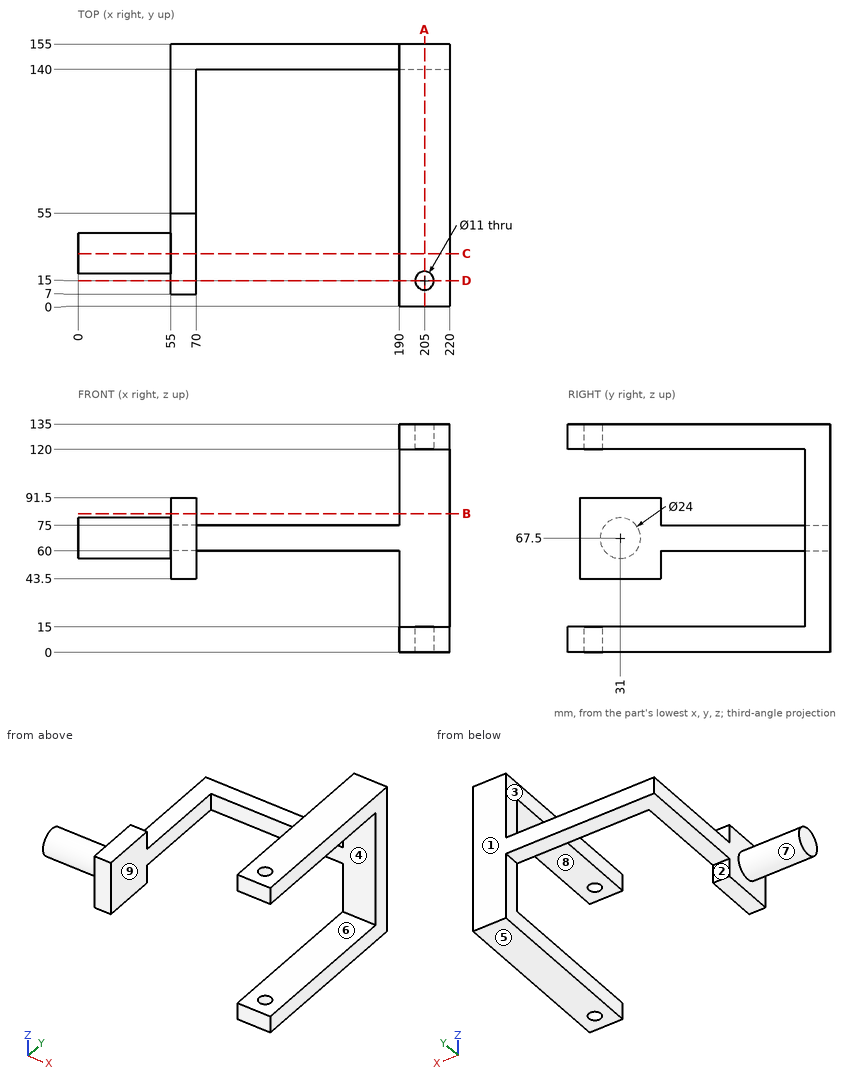
Answer from the drawing. Dimensions are ordinates in mm from the lowest x, y and z of the part. A direction names the side the tool comes from. Coordinates: 2 decimals unless noted, no trailing zeros. Loops run counter-clockwise (first coordinate to the right, second up) from the corner with the lowest first, then second, coordinate; pieces in that order, holes last. Notation, with made-up numbers: (54.25, 75.25) -> (60.25, 75.25) arc R24 cw to (60.25, 88.25) -> close; hole circle Ø11 at (-30.5, 71). An arc over 180 degrees is marked (long way). Return JSON: item names as keys, results as strings.
Item 1: Find section B-B (z = 82). Determine the outline of the cut face in (x, y), plus the area to 3 significant figures.
Answers:
{"outline": "(55, 7) -> (70, 7) -> (70, 55) -> (55, 55) -> close; (190, 140) -> (220, 140) -> (220, 155) -> (190, 155) -> close", "area": "1,170 mm2"}
Item 2: For a pull along Z with two mould halves and no side action, classify the marked faces 6, 7, 8 and 9 as +Z half, -Z half, draft (parallel to the pull), parting line (faces both ways), or undercut.
Answers:
{"face 6": "undercut", "face 7": "parting line", "face 8": "undercut", "face 9": "draft"}
Item 3: Find section D-D (y = 15). Determine the outline of the cut face in (x, z).
Answers:
{"outline": "(55, 43.5) -> (70, 43.5) -> (70, 91.5) -> (55, 91.5) -> close; (190, 0) -> (199.5, 0) -> (199.5, 15) -> (190, 15) -> close; (190, 120) -> (199.5, 120) -> (199.5, 135) -> (190, 135) -> close; (210.5, 0) -> (220, 0) -> (220, 15) -> (210.5, 15) -> close; (210.5, 120) -> (220, 120) -> (220, 135) -> (210.5, 135) -> close"}
Item 4: For the marked faces 1, 2, 3, 4 and 5, determine the directions among +Z, -Z, +X, -X, +Y, -Y from which every point of the face is accessible in a straight line to the end or side of a thin tool.
Answers:
{"face 1": "+Z, -Z, +X, -X, +Y", "face 2": "-Z, +X, -X, +Y", "face 3": "+Z, -X, +Y, -Y", "face 4": "+X, -Y", "face 5": "-Z, +X, -X, +Y, -Y"}
Item 5: Find section A-A (x = 205). Determine the outline of the cut face in (y, z).
Answers:
{"outline": "(0, 0) -> (9.5, 0) -> (9.5, 15) -> (0, 15) -> close; (0, 120) -> (9.5, 120) -> (9.5, 135) -> (0, 135) -> close; (20.5, 0) -> (155, 0) -> (155, 135) -> (20.5, 135) -> (20.5, 120) -> (140, 120) -> (140, 15) -> (20.5, 15) -> close"}
Item 6: Find the intervals of material crossed by probe 1 along Z at (x, y) = (208.5, 95.5); probe 2 along Y at (x, z) = (205, 4); probe 3 along Z at (x, y) = (103, 142), in increasing order.
Answers:
{"probe 1": "z = 0 to 15, 120 to 135", "probe 2": "y = 0 to 9.5, 20.5 to 155", "probe 3": "z = 60 to 75"}
Item 7: Find section C-C (y = 31). Determine the outline of the cut face in (x, z), plus the area to 3 significant figures.
Answers:
{"outline": "(0, 55.5) -> (55, 55.5) -> (55, 43.5) -> (70, 43.5) -> (70, 91.5) -> (55, 91.5) -> (55, 79.5) -> (0, 79.5) -> close; (190, 0) -> (220, 0) -> (220, 15) -> (190, 15) -> close; (190, 120) -> (220, 120) -> (220, 135) -> (190, 135) -> close", "area": "2,940 mm2"}
Item 8: Flat-ended cylindrical pins translate along their axes: P1, Ø10, axis at y = 18.5, z = 14, coming from the -X side; P2, Ø6.5, axis at x = 205, y = 15, coming from the -Z side; P3, Ø4.5, axis at x = 64.5, y = 22.5, coming from the -Z side; P4, Ø4.5, axis at x = 64.5, y = 42.5, coming from the +Z side. Find the tip coordinate at first contact, or state that the pin passes through.
Answers:
{"P1": "stops at x = 190", "P2": "passes through", "P3": "stops at z = 43.5", "P4": "stops at z = 91.5"}
